Check sheet for the modelled part. Datum: model origin and axes. Units: mm. Face numbers are marked on the shaded views. Coordinates: 2 decimals unless noted, no trailing zeros. Write each loop counter-clockwise with the first axis right and the second up, starting at its lowest first coordinate (ties: lowest second). Pieces come first, ordered by that corner, then holes. Notation, with made-up numbers: (72.25, 0.5) -> (77.25, 0.5) arc R15 cw to (77.25, 24.5) -> close; hole circle Ø2 at (31.5, -27.75). An arc over 180 degrees is marked (long way). Put each result on its own line as item: value.
```python
from build123d import *

# Parameters (mm, degrees)
BOSS_EXTRUDE2_DEPTH                          = 3
SKETCH4_W                                    = 50
SKETCH4_H                                    = 15
BOSS_EXTRUDE3_DEPTH                          = 3
SKETCH6_R                                    = 5
BOSS_EXTRUDE4_DEPTH                          = 5
FILLET1_R                                    = 5
FILLET2_R                                    = 5
CSK_FOR_M4_COUNTERSUNK_FLAT_HEAD_SCR_2_COUNT = 2
CSK_FOR_M4_COUNTERSUNK_FLAT_HEAD_SCR_2_PITCH = 16
CSK_FOR_M4_COUNTERSUNK_FLAT_HEAD_SCR_3_COUNT = 2
CSK_FOR_M4_COUNTERSUNK_FLAT_HEAD_SCR_3_PITCH = 16
SKETCH9_R                                    = 1.175
CUT_EXTRUDE2_DEPTH                           = 49.125772869
CHAMFER1_SIZE                                = 2.5


with BuildPart() as part:
    # Sketch2 → Boss-Extrude2 (new body)
    with BuildSketch(Plane(origin=(0, 0, 0), x_dir=(1, 0, 0), z_dir=(0, 1, 0))):
        with BuildLine():
            Line((-35.700010115, -20.037625203), (19.399989885, 5.462374797))
            ThreePointArc((19.399989885, 5.462374797), (21.837625203, 12.099989885), (15.200010115, 14.537625203))
            Line((15.200010115, 14.537625203), (-39.899989885, -10.962374797))
            ThreePointArc((-39.899989885, -10.962374797), (-42.337625203, -17.599989885), (-35.700010115, -20.037625203))
        make_face()
    extrude(amount=BOSS_EXTRUDE2_DEPTH)

    # Sketch4 → Boss-Extrude3 (add)
    with BuildSketch(Plane(origin=(0, 0, 0), x_dir=(1, 0, 0), z_dir=(0, 1, 0))):
        Rectangle(SKETCH4_W, SKETCH4_H)
    extrude(amount=BOSS_EXTRUDE3_DEPTH)

    # Sketch6 → Boss-Extrude4 (add)
    with BuildSketch(Plane(origin=(0, 3, 0), x_dir=(1, 0, 0), z_dir=(0, 1, 0))):
        with Locations(Location((-37.8, -15.5, 0), (0, 0, 114.834459772))):
            Circle(SKETCH6_R)
        with Locations(Location((17.3, 10, 0), (0, 0, 114.834459772))):
            Circle(SKETCH6_R)
    extrude(amount=BOSS_EXTRUDE4_DEPTH)

    # Fillet1
    # the kernel refuses this fillet: 5 mm, written as the material it adds along each edge
    with BuildSketch(Plane(origin=(-25, 0, 4.066735195), x_dir=(0, 0, -1), z_dir=(0, 1, 0))) as fillet1_piece_1:
        with BuildLine():
            CenterArc((FILLET1_R * 0.639103051734, FILLET1_R), FILLET1_R, 204.834459772, 65.165540228)
            Line((-FILLET1_R * 0.268421988848, FILLET1_R * 0.580002022961), (0, 0))
            Line((0, 0), (FILLET1_R * 0.639103051734, 0))
        make_face()
    extrude(amount=3)
    with BuildSketch(Plane(origin=(-0.00678003, 3, -7.5), x_dir=(0.9075250405819563, 0, -0.419997977038841), z_dir=(0, -1, 0)), Plane(origin=(-8.608906245, 3, 7.5), x_dir=(-0.9075250405819576, 0, 0.41999797703883784), z_dir=(0, -1, 0))) as fillet1_piece_2:
        with BuildLine():
            CenterArc((FILLET1_R * 0.220179535316, -FILLET1_R), FILLET1_R, 90, 24.834459772)
            Line((-FILLET1_R * 0.199818441723, -FILLET1_R * 0.092474959418), (0, 0))
            Line((0, 0), (FILLET1_R * 0.220179535316, 0))
        make_face()
    extrude(amount=3)
    # the kernel refuses this fillet: 5 mm, written as the material it takes off along each edge
    with BuildSketch(Plane(origin=(25, -11.817012604, -7.5), x_dir=(0, 0, 1), z_dir=(0, 1, 0))) as fillet1_2_piece_1:
        with BuildLine():
            CenterArc((4.726805042, -5), FILLET1_R, 90, 70.972289662)
            Line((0, -3.369872981), (0, 0))
            Line((0, 0), (4.726805042, 0))
        make_face()
    extrude(amount=26.634025208, mode=Mode.SUBTRACT)
    with BuildSketch(Plane(origin=(-25, -12.5, -7.5), x_dir=(1, 0, 0), z_dir=(0, 1, 0)), Plane(origin=(25, -12.5, 7.5), x_dir=(-1, 0, 0), z_dir=(0, 1, 0))) as fillet1_2_piece_2:
        with BuildLine():
            CenterArc((FILLET1_R, -FILLET1_R), FILLET1_R, 90, 90)
            Line((0, -FILLET1_R), (0, 0))
            Line((0, 0), (FILLET1_R, 0))
        make_face()
    extrude(amount=28, mode=Mode.SUBTRACT)

    # Fillet2
    fillet2_edges = [part.edges().sort_by_distance(p)[0] for p in [
        (21.630127019, 1.5, -7.5),
    ]]
    fillet(fillet2_edges, radius=FILLET2_R)

    # Sketch7 → CSK for M4 Countersunk Flat Head Screw1 (revolve, cut)
    with BuildSketch(Plane(origin=(0, 3, 0), x_dir=(0, 0, 1), z_dir=(1, 0, 0))):
        Polygon((0, 0), (0, 3.000025), (2.25, 3.000025), (2.25, 2.45), (4.7, 0), align=None)
    csk_for_m4_countersunk_flat_head_screw1 = revolve(axis=Axis((0, 9.35, 0), (0, -1, 0)), mode=Mode.SUBTRACT)

    # CSK for M4 Countersunk Flat Head Scr 2: CSK for M4 Countersunk Flat Head Screw1 ×2
    with Locations(*[(-i * CSK_FOR_M4_COUNTERSUNK_FLAT_HEAD_SCR_2_PITCH, 0, 0) for i in range(1, CSK_FOR_M4_COUNTERSUNK_FLAT_HEAD_SCR_2_COUNT)]):
        add(csk_for_m4_countersunk_flat_head_screw1, mode=Mode.SUBTRACT)

    # CSK for M4 Countersunk Flat Head Scr 3: CSK for M4 Countersunk Flat Head Screw1 ×2
    with Locations(*[(i * CSK_FOR_M4_COUNTERSUNK_FLAT_HEAD_SCR_3_PITCH, 0, 0) for i in range(1, CSK_FOR_M4_COUNTERSUNK_FLAT_HEAD_SCR_3_COUNT)]):
        add(csk_for_m4_countersunk_flat_head_screw1, mode=Mode.SUBTRACT)

    # Sketch9 → Cut-Extrude2 (cut, through all)
    with BuildSketch(Plane(origin=(0, 8, 0), x_dir=(1, 0, 0), z_dir=(0, 1, 0))):
        with Locations(Location((-37.8, -15.5, 0), (0, 0, 270))):
            Circle(SKETCH9_R)
        with Locations(Location((17.3, 10, 0), (0, 0, 270))):
            Circle(SKETCH9_R)
    extrude(amount=-CUT_EXTRUDE2_DEPTH, mode=Mode.SUBTRACT)

    # Chamfer1
    chamfer1_edges = [part.edges().sort_by_distance(p)[0] for p in [
        (-35.700010115, 8, 20.037625203),
        (19.399989885, 8, -5.462374797),
    ]]
    chamfer(chamfer1_edges, length=CHAMFER1_SIZE)


solid = part.part
```
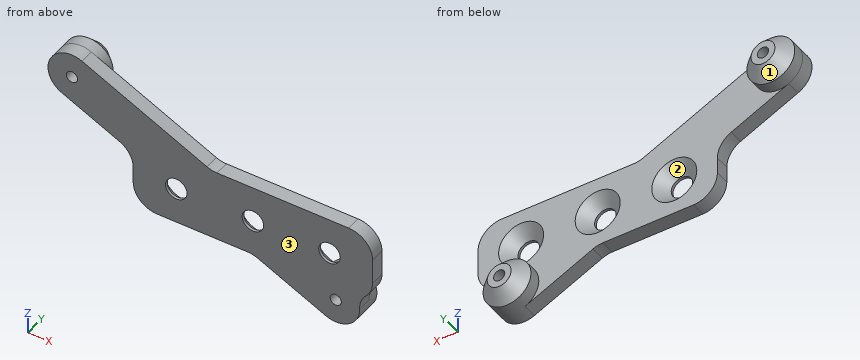
Q1. Mould release check, pull along X, two halves, no side actions. Record for the marked faces 1, 2 and 3: released by +X, released by -X, zero draft, split by the parting line, or undercut.
Recorded:
face 1: split by the parting line
face 2: undercut
face 3: zero draft
Q2. Cross-section at C-C (x = -37.8). Record the cut outline in (y, z) (3 decimals), plus the area to 3 significant figures.
Recorded:
outline: (0, 9.991) -> (3, 9.991) -> (3, 10.5) -> (5.5, 10.5) -> (8, 13) -> (8, 14.325) -> (0, 14.325) -> close; (0, 16.675) -> (8, 16.675) -> (8, 18) -> (5.5, 20.5) -> (0, 20.5) -> close
area: 56.5 mm2
Q3. Material ranges on line 1 along X through (y, z) = (0.2, 0); line 2 along X through (y, z) = (2.25, -10) (3 decimals); line 3 along Y through (x, z) = (-20.5, -4), recorded low to high.
Recorded:
line 1: x = -25 to -18.25, -13.75 to -2.25, 2.25 to 13.75, 18.25 to 25
line 2: x = 5.395 to 16.125, 18.475 to 22.3
line 3: y = 0 to 3
Q4. Cross-section at B-B (y = 3.75). Record the cut outline in (x, z) (3 decimals), plus the area to 3 significant figures.
Recorded:
outline: circle Ø10 at (-37.8, 15.5); circle Ø10 at (17.3, -10); hole circle Ø2.35 at (-37.8, 15.5); hole circle Ø2.35 at (17.3, -10)
area: 148 mm2
Q5. Cross-section at D-D (z = 15.5). Record the cut outline in (x, y) (3 decimals).
Recorded:
outline: (-42.8, 0) -> (-38.975, 0) -> (-38.975, 8) -> (-40.3, 8) -> (-42.8, 5.5) -> close; (-36.625, 0) -> (-25.895, 0) -> (-25.895, 3) -> (-32.8, 3) -> (-32.8, 5.5) -> (-35.3, 8) -> (-36.625, 8) -> close
Q6. Depth check by flat-ended pin: P1, Ø3, axis at x = -4.5, z = 4, coming from the -Y side; P2, Ø0.9, axis at x = -11.5, y = 1, coming from the -Z side; P3, Ø2, axis at x = 17.3, z = -10, coming from the -Y side; P4, Ø8, axis at x = -5, z = -9, coming from the +Y side. Enter the tip coordinate at first touch or a pass-through.
Recorded:
P1: stops at y = 0
P2: stops at z = -7.5
P3: passes through
P4: stops at y = 3
Q7. Cross-section at A-A (z = 0). Record the cut outline in (x, y).
Recorded:
outline: (-25, 0) -> (-18.25, 0) -> (-18.25, 0.55) -> (-20.7, 3) -> (-25, 3) -> close; (-13.75, 0) -> (-2.25, 0) -> (-2.25, 0.55) -> (-4.7, 3) -> (-11.3, 3) -> (-13.75, 0.55) -> close; (2.25, 0) -> (13.75, 0) -> (13.75, 0.55) -> (11.3, 3) -> (4.7, 3) -> (2.25, 0.55) -> close; (18.25, 0) -> (25, 0) -> (25, 3) -> (20.7, 3) -> (18.25, 0.55) -> close
